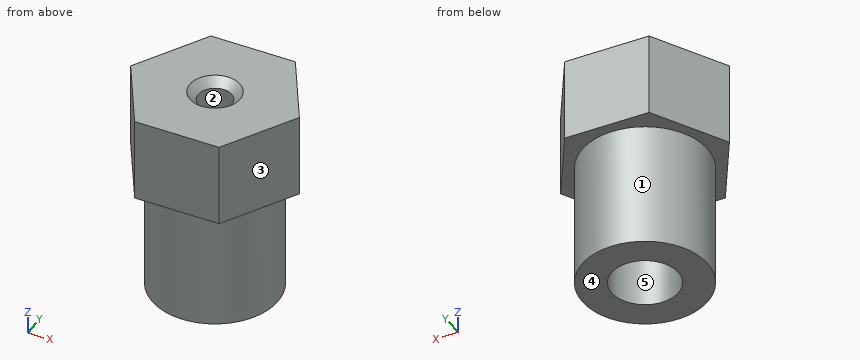
```python
from build123d import *

# Parameters (mm, degrees)
SKETCH1_R           = 4.7625
SKETCH1_R_2         = 2.54
BOSS_EXTRUDE1_DEPTH = 9.525
BOSS_EXTRUDE2_DEPTH = 6.35
CUT_EXTRUDE1_REACH  = 17.875
SKETCH3_R           = 1.27
CHAMFER1_SIZE       = 0.635


with BuildPart() as part:
    # Sketch1 → Boss-Extrude1 (new body)
    with BuildSketch(Plane.XY):
        Circle(SKETCH1_R)
        Circle(SKETCH1_R_2, mode=Mode.SUBTRACT)
    extrude(amount=BOSS_EXTRUDE1_DEPTH)

    # Sketch2 → Boss-Extrude2 (add)
    with BuildSketch(Plane.XY.offset(9.525)):
        Polygon((3.022954056, 5.659001754), (-3.389362251, 5.447455885), (-6.412316308, -0.21154587), (-3.022954056, -5.659001754), (3.389362251, -5.447455885), (6.412316308, 0.21154587), align=None)
    extrude(amount=BOSS_EXTRUDE2_DEPTH)

    # Sketch3 → Cut-Extrude1 (cut, up to next)
    with BuildSketch(Plane.XY.offset(15.875), mode=Mode.PRIVATE) as cut_extrude1_sk1:
        Circle(SKETCH3_R)
    cut_extrude1_tool1 = extrude(cut_extrude1_sk1.sketch, amount=-CUT_EXTRUDE1_REACH, mode=Mode.PRIVATE) & part.part
    add(cut_extrude1_tool1.solids().sort_by_distance((0, 0, 15.875))[0], mode=Mode.SUBTRACT)

    # Chamfer1
    chamfer1_edges = [part.edges().sort_by_distance(p)[0] for p in [
        (-1.27, 0, 15.875),
    ]]
    chamfer(chamfer1_edges, length=CHAMFER1_SIZE)


solid = part.part
```
The model under review builds one solid part; all positions refer to its coordinate system, in mm. Face numbers are marked on the shaded views. A direction names the side the tool comes from. Round coordinates to 2 decimals unless told otherwise and drop trailing zeros. Loops run counter-clockwise (first coordinate to the right, second up) from the corner with the lowest first, then second, coordinate; pieces in that order, holes last.
Item 1: Take a section at C-C (z = 4). Write out the cut boundary in (x, y) (1 decimal), then the cut area to 3 significant figures.
Determined:
outline: circle Ø9.5 at (0, 0); hole circle Ø5.1 at (0, 0)
area: 51.0 mm2
Item 2: Clearance check with flat-ended pins moving along their axes: pin 1 Ø3 at (x, z) = (0.5, 6) entering from +Y; pin 2 Ø5.5 at (x, y) = (1, -0.5) entering from -Z; pin 3 Ø1.5 at (x, y) = (0, 0) entering from -Z; pin 4 Ø4 at (y, z) = (2.5, 2) entering from +X. State where each tip first meets the part, or that it passes through.
Determined:
pin 1: stops at y = 4.76
pin 2: stops at z = 0
pin 3: passes through
pin 4: stops at x = 4.74
Item 3: For the marked faces 4 and 5, list the 3-axis set-ups (+Z, -Z, +X, -X, +Y, -Y) from which the entire face can be reached by the end or side of a thin tool; tool diameter is ignored.
Determined:
face 4: -Z, +X, -X, +Y, -Y
face 5: -Z
Item 4: Take a section at B-B (y = 0). Write out the cut boundary in (x, z) (1 decimal).
Determined:
outline: (-6.3, 9.5) - (-4.8, 9.5) - (-4.8, 0) - (-2.5, 0) - (-2.5, 9.5) - (-1.3, 9.5) - (-1.3, 15.2) - (-1.9, 15.9) - (-6.3, 15.9) - close; (1.3, 9.5) - (2.5, 9.5) - (2.5, 0) - (4.8, 0) - (4.8, 9.5) - (6.3, 9.5) - (6.3, 15.9) - (1.9, 15.9) - (1.3, 15.2) - close
Item 5: For line 1 (Y direction, x = 0, z = 4.25); line 2 (Z direction, x = -4.5, y = -2.5) (3 decimals); line 3 (Y direction, x = -0.5, z = 2), list the stretches that pass through material, from the lowest coordinate up.
Determined:
line 1: y = -4.76 to -2.54, 2.54 to 4.76
line 2: z = 9.525 to 15.875
line 3: y = -4.74 to -2.49, 2.49 to 4.74
Item 6: Take a section at A-A (x = 0). Write out the cut boundary in (y, z) (1 decimal).
Determined:
outline: (-5.6, 9.5) - (-4.8, 9.5) - (-4.8, 0) - (-2.5, 0) - (-2.5, 9.5) - (-1.3, 9.5) - (-1.3, 15.2) - (-1.9, 15.9) - (-5.6, 15.9) - close; (1.3, 9.5) - (2.5, 9.5) - (2.5, 0) - (4.8, 0) - (4.8, 9.5) - (5.6, 9.5) - (5.6, 15.9) - (1.9, 15.9) - (1.3, 15.2) - close
Item 7: Take a section at D-D (x = 4.5). Write out the cut boundary in (y, z) (3 decimals).
Determined:
outline: (-3.368, 9.525) - (-1.559, 9.525) - (-1.559, 0) - (1.559, 0) - (1.559, 9.525) - (3.285, 9.525) - (3.285, 15.875) - (-3.368, 15.875) - close
Item 8: Mouldability with a two-part tool opening along X and no side actions: class the marked faces 1, 2 and 3 as released by +X, released by -X, zero draft, split by the parting line, or undercut.
Determined:
face 1: split by the parting line
face 2: undercut
face 3: released by +X
